from build123d import *

# Parameters (mm, degrees)
SZKIC1_R                         = 72.5
DODANIE_WYCI_GNI_CIE1_DEPTH      = 5
DODANIE_WYCI_GNI_CIE2_START      = 5
SZKIC1_3_R                       = 65
SZKIC1_3_R_2                     = 54.5
DODANIE_WYCI_GNI_CIE2_DEPTH      = 8
DODANIE_WYCI_GNI_CIE3_START      = 13
SZKIC1_4_R                       = 54.5
DODANIE_WYCI_GNI_CIE3_DEPTH      = 30
DODANIE_WYCI_GNI_CIE4_START      = 43
SZKIC2_W                         = 34
SZKIC2_H                         = 88
DODANIE_WYCI_GNI_CIE4_DEPTH      = 93
SZKIC3_R                         = 45
WYTNIJ_WYCI_GNI_CIE1_DEPTH       = 10
DODANIE_WYCI_GNI_CIE5_START      = 10
SZKIC4_R                         = 3
DODANIE_WYCI_GNI_CIE5_DEPTH      = 13
ZAAWANSOWANYOTW_R1_OUTLINE_R     = 1.75
ZAAWANSOWANYOTW_R1_DEPTH         = 13
ZAAWANSOWANYOTW_R1_START         = 10
ZAAWANSOWANYOTW_R1_2_OUTLINE_R   = 3
ZAAWANSOWANYOTW_R1_2_OUTLINE_R_2 = 1.75
ZAAWANSOWANYOTW_R1_2_DEPTH       = 3
SZKIC7_R                         = 4.25
WYTNIJ_WYCI_GNI_CIE2_START       = -13
WYTNIJ_WYCI_GNI_CIE2_DEPTH       = 3.5
PRZECI_CIE1_START                = 5
PRZECI_CIE1_OUTLINE_R            = 1.75
PRZECI_CIE1_DEPTH                = 131
PRZECI_CIE1_START_2              = -3
PRZECI_CIE1_2_OUTLINE_R          = 3
PRZECI_CIE1_2_DEPTH              = 8


# Read off the part's stored shape, not the designer's step: ZaawansowanyOtwór1, Przecięcie1
with BuildPart() as part:
    # Szkic1 → Dodanie-wyciągnięcie1 (new body)
    with BuildSketch(Plane(origin=(0, 0, 0), x_dir=(1, 0, 0), z_dir=(0, 1, 0))):
        with Locations(Location((0, 0, 0), (0, 0, 270))):
            Circle(SZKIC1_R)
    extrude(amount=DODANIE_WYCI_GNI_CIE1_DEPTH)

    # Szkic1<3> → Dodanie-wyciągnięcie2 (add)
    with BuildSketch(Plane(origin=(0, 0, 0), x_dir=(1, 0, 0), z_dir=(0, 1, 0)).offset(DODANIE_WYCI_GNI_CIE2_START)):
        with Locations(Location((0, 0, 0), (0, 0, 270))):
            Circle(SZKIC1_3_R)
        Circle(SZKIC1_3_R_2)
    extrude(amount=DODANIE_WYCI_GNI_CIE2_DEPTH)

    # Szkic1<4> → Dodanie-wyciągnięcie3 (add)
    with BuildSketch(Plane(origin=(0, 0, 0), x_dir=(1, 0, 0), z_dir=(0, 1, 0)).offset(DODANIE_WYCI_GNI_CIE3_START)):
        with Locations(Location((0, 0, 0), (0, 0, 270))):
            Circle(SZKIC1_4_R)
    extrude(amount=DODANIE_WYCI_GNI_CIE3_DEPTH)

    # Szkic2 → Dodanie-wyciągnięcie4 (add)
    with BuildSketch(Plane(origin=(0, 0, 0), x_dir=(1, 0, 0), z_dir=(0, 1, 0)).offset(DODANIE_WYCI_GNI_CIE4_START)):
        with Locations((-44.5, -12.5)):
            Rectangle(SZKIC2_W, SZKIC2_H)
        with Locations((44.5, -12.5)):
            Rectangle(SZKIC2_W, SZKIC2_H)
    extrude(amount=DODANIE_WYCI_GNI_CIE4_DEPTH)

    # Szkic3 → Wytnij-wyciągnięcie1 (cut)
    with BuildSketch(Plane(origin=(0, 0, 0), x_dir=(1, 0, 0), z_dir=(0, 1, 0))):
        with Locations(Location((0, 0, 0), (0, 0, 270))):
            Circle(SZKIC3_R)
    extrude(amount=WYTNIJ_WYCI_GNI_CIE1_DEPTH, mode=Mode.SUBTRACT)

    # Szkic4 → Dodanie-wyciągnięcie5 (add)
    with BuildSketch(Plane(origin=(0, 0, 0), x_dir=(1, 0, 0), z_dir=(0, 1, 0)).offset(DODANIE_WYCI_GNI_CIE5_START)):
        with Locations(Location((0, 0, 0), (0, 0, 270))):
            Circle(SZKIC4_R)
    extrude(amount=-DODANIE_WYCI_GNI_CIE5_DEPTH)

    # ZaawansowanyOtwór1 outline → ZaawansowanyOtwór1 (cut)
    with BuildSketch(Plane(origin=(0, 0, 0), x_dir=(1, 0, 0), z_dir=(0, 1, 0))):
        with Locations((-42.391051532, 42.391051532)):
            Circle(ZAAWANSOWANYOTW_R1_OUTLINE_R)
        with Locations((-59.95, 0)):
            Circle(ZAAWANSOWANYOTW_R1_OUTLINE_R)
        with Locations((-42.391051532, -42.391051532)):
            Circle(ZAAWANSOWANYOTW_R1_OUTLINE_R)
        with Locations((0, -59.95)):
            Circle(ZAAWANSOWANYOTW_R1_OUTLINE_R)
        with Locations((42.391051532, -42.391051532)):
            Circle(ZAAWANSOWANYOTW_R1_OUTLINE_R)
        with Locations((59.95, 0)):
            Circle(ZAAWANSOWANYOTW_R1_OUTLINE_R)
        with Locations((42.391051532, 42.391051532)):
            Circle(ZAAWANSOWANYOTW_R1_OUTLINE_R)
        with Locations((0, 59.95)):
            Circle(ZAAWANSOWANYOTW_R1_OUTLINE_R)
    extrude(amount=ZAAWANSOWANYOTW_R1_DEPTH, mode=Mode.SUBTRACT)

    # ZaawansowanyOtw_r1 2 outline → ZaawansowanyOtw_r1 2 (cut)
    # profile 1 of 8: a face of its own
    with BuildSketch(Plane(origin=(0, 0, 0), x_dir=(1, 0, 0), z_dir=(0, 1, 0)).offset(ZAAWANSOWANYOTW_R1_START)):
        with Locations((-42.391051532, 42.391051532)):
            Circle(ZAAWANSOWANYOTW_R1_2_OUTLINE_R)
        with Locations((-42.391051532, 42.391051532)):
            Circle(ZAAWANSOWANYOTW_R1_2_OUTLINE_R_2, mode=Mode.SUBTRACT)
    # profile 2 of 8: a face of its own
    with BuildSketch(Plane(origin=(0, 0, 0), x_dir=(1, 0, 0), z_dir=(0, 1, 0)).offset(ZAAWANSOWANYOTW_R1_START)):
        with Locations((-59.95, 0)):
            Circle(ZAAWANSOWANYOTW_R1_2_OUTLINE_R)
        with Locations((-59.95, 0)):
            Circle(ZAAWANSOWANYOTW_R1_2_OUTLINE_R_2, mode=Mode.SUBTRACT)
    # profile 3 of 8: a face of its own
    with BuildSketch(Plane(origin=(0, 0, 0), x_dir=(1, 0, 0), z_dir=(0, 1, 0)).offset(ZAAWANSOWANYOTW_R1_START)):
        with Locations((-42.391051532, -42.391051532)):
            Circle(ZAAWANSOWANYOTW_R1_2_OUTLINE_R)
        with Locations((-42.391051532, -42.391051532)):
            Circle(ZAAWANSOWANYOTW_R1_2_OUTLINE_R_2, mode=Mode.SUBTRACT)
    # profile 4 of 8: a face of its own
    with BuildSketch(Plane(origin=(0, 0, 0), x_dir=(1, 0, 0), z_dir=(0, 1, 0)).offset(ZAAWANSOWANYOTW_R1_START)):
        with Locations((0, -59.95)):
            Circle(ZAAWANSOWANYOTW_R1_2_OUTLINE_R)
        with Locations((0, -59.95)):
            Circle(ZAAWANSOWANYOTW_R1_2_OUTLINE_R_2, mode=Mode.SUBTRACT)
    # profile 5 of 8: a face of its own
    with BuildSketch(Plane(origin=(0, 0, 0), x_dir=(1, 0, 0), z_dir=(0, 1, 0)).offset(ZAAWANSOWANYOTW_R1_START)):
        with Locations((42.391051532, -42.391051532)):
            Circle(ZAAWANSOWANYOTW_R1_2_OUTLINE_R)
        with Locations((42.391051532, -42.391051532)):
            Circle(ZAAWANSOWANYOTW_R1_2_OUTLINE_R_2, mode=Mode.SUBTRACT)
    # profile 6 of 8: a face of its own
    with BuildSketch(Plane(origin=(0, 0, 0), x_dir=(1, 0, 0), z_dir=(0, 1, 0)).offset(ZAAWANSOWANYOTW_R1_START)):
        with Locations((59.95, 0)):
            Circle(ZAAWANSOWANYOTW_R1_2_OUTLINE_R)
        with Locations((59.95, 0)):
            Circle(ZAAWANSOWANYOTW_R1_2_OUTLINE_R_2, mode=Mode.SUBTRACT)
    # profile 7 of 8: a face of its own
    with BuildSketch(Plane(origin=(0, 0, 0), x_dir=(1, 0, 0), z_dir=(0, 1, 0)).offset(ZAAWANSOWANYOTW_R1_START)):
        with Locations((42.391051532, 42.391051532)):
            Circle(ZAAWANSOWANYOTW_R1_2_OUTLINE_R)
        with Locations((42.391051532, 42.391051532)):
            Circle(ZAAWANSOWANYOTW_R1_2_OUTLINE_R_2, mode=Mode.SUBTRACT)
    # profile 8 of 8: a face of its own
    with BuildSketch(Plane(origin=(0, 0, 0), x_dir=(1, 0, 0), z_dir=(0, 1, 0)).offset(ZAAWANSOWANYOTW_R1_START)):
        with Locations((0, 59.95)):
            Circle(ZAAWANSOWANYOTW_R1_2_OUTLINE_R)
        with Locations((0, 59.95)):
            Circle(ZAAWANSOWANYOTW_R1_2_OUTLINE_R_2, mode=Mode.SUBTRACT)
    extrude(amount=ZAAWANSOWANYOTW_R1_2_DEPTH, mode=Mode.SUBTRACT)

    # Szkic7 → Wycięcie-obrót1 (revolve, cut)
    with BuildSketch(Plane(origin=(0, 0, 0), x_dir=(0, 0, -1), z_dir=(1, 0, 0)), mode=Mode.PRIVATE) as wyci_cie_obr_t1_sk:
        with Locations((51, -1.7)):
            Circle(SZKIC7_R)
    revolve(wyci_cie_obr_t1_sk.sketch.rotate(Axis((0, 0, 0), (0, -1, 0)), 305.308707607), axis=Axis((0, 0, 0), (0, -1, 0)), mode=Mode.SUBTRACT)

    # Szkic5 → Wytnij-wyciągnięcie2 (cut)
    with BuildSketch(Plane(origin=(0, 13, 0), x_dir=(1, 0, 0), z_dir=(0, 1, 0)).offset(WYTNIJ_WYCI_GNI_CIE2_START)):
        Polygon((43.227855306, 39.268057332), (45.514045733, 41.554247758), (44.677241959, 44.677241959), (41.554247758, 45.514045733), (39.268057332, 43.227855306), (40.104861106, 40.104861106), align=None)
        Polygon((-2.8, 61.566580754), (-2.8, 58.333419246), (0, 56.716838493), (2.8, 58.333419246), (2.8, 61.566580754), (0, 63.183161507), align=None)
        Polygon((58.333419246, -2.8), (61.566580754, -2.8), (63.183161507, 0), (61.566580754, 2.8), (58.333419246, 2.8), (56.716838493, 0), align=None)
        Polygon((39.268057332, -43.227855306), (41.554247758, -45.514045733), (44.677241959, -44.677241959), (45.514045733, -41.554247758), (43.227855306, -39.268057332), (40.104861106, -40.104861106), align=None)
        Polygon((-2.8, -58.333419246), (-2.8, -61.566580754), (0, -63.183161507), (2.8, -61.566580754), (2.8, -58.333419246), (0, -56.716838493), align=None)
        Polygon((-43.227855306, -39.268057332), (-45.514045733, -41.554247758), (-44.677241959, -44.677241959), (-41.554247758, -45.514045733), (-39.268057332, -43.227855306), (-40.104861106, -40.104861106), align=None)
        Polygon((-58.333419246, 2.8), (-61.566580754, 2.8), (-63.183161507, 0), (-61.566580754, -2.8), (-58.333419246, -2.8), (-56.716838493, 0), align=None)
        Polygon((-39.268057332, 43.227855306), (-41.554247758, 45.514045733), (-44.677241959, 44.677241959), (-45.514045733, 41.554247758), (-43.227855306, 39.268057332), (-40.104861106, 40.104861106), align=None)
    extrude(amount=WYTNIJ_WYCI_GNI_CIE2_DEPTH, mode=Mode.SUBTRACT)

    # Przecięcie1 outline → Przecięcie1 (cut)
    with BuildSketch(Plane(origin=(0, 0, 0), x_dir=(1, 0, 0), z_dir=(0, 1, 0)).offset(PRZECI_CIE1_START)):
        with BuildLine():
            ThreePointArc((61.5, -21.041625412), (65, 0), (61.5, 21.041625413))
            Line((61.5, 21.041625413), (61.5, 31.5))
            Line((61.5, 31.5), (56.857277459, 31.5))
            ThreePointArc((56.857277459, 31.5), (0, 65), (-56.857277459, 31.5))
            Line((-56.857277459, 31.5), (-61.5, 31.5))
            Line((-61.5, 31.5), (-61.5, 21.041625412))
            ThreePointArc((-61.5, 21.041625412), (-65, 0), (-61.5, -21.041625412))
            Line((-61.5, -21.041625412), (-61.5, -56.5))
            Line((-61.5, -56.5), (-32.136427928, -56.5))
            ThreePointArc((-32.136427928, -56.5), (0, -65), (32.136427928, -56.5))
            Line((32.136427928, -56.5), (61.5, -56.5))
            Line((61.5, -56.5), (61.5, -21.041625412))
        make_face()
        with BuildLine():
            ThreePointArc((61.5, 0.81240384), (61.7, 0), (61.5, -0.81240384))
            Line((61.5, -0.81240384), (61.5, 0.81240384))
        make_face(mode=Mode.SUBTRACT)
        with Locations((0, -59.95)):
            Circle(PRZECI_CIE1_OUTLINE_R, mode=Mode.SUBTRACT)
        with Locations((42.391051532, 42.391051532)):
            Circle(PRZECI_CIE1_OUTLINE_R, mode=Mode.SUBTRACT)
        with Locations((-42.391051532, 42.391051532)):
            Circle(PRZECI_CIE1_OUTLINE_R, mode=Mode.SUBTRACT)
        with Locations((0, 59.95)):
            Circle(PRZECI_CIE1_OUTLINE_R, mode=Mode.SUBTRACT)
        with BuildLine():
            ThreePointArc((-61.5, -0.81240384), (-61.7, 0), (-61.5, 0.81240384))
            Line((-61.5, 0.81240384), (-61.5, -0.81240384))
        make_face(mode=Mode.SUBTRACT)
    extrude(amount=PRZECI_CIE1_DEPTH, mode=Mode.SUBTRACT)

    # Przeci_cie1 2 outline → Przeci_cie1 2 (cut)
    with BuildSketch(Plane(origin=(0, 0, 0), x_dir=(1, 0, 0), z_dir=(0, 1, 0)).offset(PRZECI_CIE1_START_2)):
        Circle(PRZECI_CIE1_2_OUTLINE_R)
    extrude(amount=PRZECI_CIE1_2_DEPTH, mode=Mode.SUBTRACT)


solid = part.part
Part model, mm, in its own coordinate system. A direction names the side the tool comes from. Coordinates: 2 decimals unless noted, no trailing zeros. Write each question's results on one line, items separated by ' | '. Start each with the question number.
Q1. Which spindle directions (+Z, -Z, +X, -X, +Y, -Y) get a long thin tool onto all of the face, cutting with end or side? Do faces 1 (the flat face through (41, 3.5, -41)), 2 (the cylindrical face through (-43.681, 4.24, -43.574)). Say none if no direction does.
Q2. Probe line 1 along X through (y, z) = (0.4, -9.5); line 2 along Z through (x, y) = (0.5, 3.3); line 3 along Z through (x, y) = (-29, 1.55). List the from-to ranges inside material, lowest first.
Q3. Two-plate mould, pull along Z, no slides. Class faces 3 (the flat face through (-24.2, 0, 38.2)), 4 (the flat face through (60, 2, -2.8)): +Z half, -Z half, draft (parallel to the pull), parting line (faces both ways), or undercut.
Q4. Drop flat-ended pins along their axis: pin 1 Ø2 at (x, y) = (-49, 1) entering from -Z; pin 2 Ø3 at (x, z) = (43, 43) entering from -Y; pin 3 Ø1 at (x, y) = (59.5, 1) entering from +Z; pin 4 Ø6 at (x, z) = (0.5, 61) entering from -Y. Give the stop position or say it passes through.
Q5. Slice it at A-A on y = 1.25. Give the number of separate pieces and of enclosed holes in the cut face, and give its area (3 significant figures).
Answer:
1) face 1: -Y | face 2: +Y, -Y
2) line 1: x = -71.87 to -53.86, -46.34 to -43.99, 43.99 to 46.34, 53.86 to 71.87 | line 2: z = -72.5 to -62.89, -57.01 to -45, 45 to 57.01, 62.89 to 72.5 | line 3: z = -66.45 to -45.24, -38.58 to -34.41, 34.41 to 38.58, 45.24 to 66.45
3) face 3: draft | face 4: undercut
4) pin 1: stops at z = -54.33 | pin 2: stops at y = 3.5 | pin 3: stops at z = 42.13 | pin 4: stops at y = 0
5) separate pieces: 2 | enclosed holes: 10 | area: 7,970 mm2
